Read the model definition and answer for the solid it produces. Units are mm, in the model's axes. A direction names the side the tool comes from. Coordinates: 2 decimals unless noted, no trailing zeros. Write each loop counter-clockwise with the first axis right and the second up, starting at its lowest first coordinate (ties: lowest second). Pieces come first, ordered by that corner, then holes. Notation, with made-up numbers: (67, 17.5) -> (119, 17.5) arc R10 ccw to (119, 31.5) -> close; hole circle Ø4 at (87.25, 79). An arc over 180 degrees is marked (long way). Use CSV: the item, a comma, the result in double quotes.
from build123d import *

# Parameters (mm, degrees)
F1_DEPTH = 5
F3_DEPTH = 2
F5_R     = 4.0386
F6_DEPTH = 2


with BuildPart() as f1:
    # F0 (on Top) → F1 (new body)
    with BuildSketch(Plane.XY):
        with BuildLine():
            ThreePointArc((-26.651348, 17.408332), (-28.98701, 16.85103), (-31.313855, 16.257994))
            Line((-31.313855, 16.257994), (-31.313855, -1.454417))
            ThreePointArc((-31.313855, -1.454417), (-29.445548, -2.127472), (-27.565881, -2.768118))
            Line((-27.565881, -2.768118), (-27.565881, 8.0386))
            Line((-27.565881, 8.0386), (-23.981268, -3.890644))
            ThreePointArc((-23.981268, -3.890644), (-21.785328, -4.515397), (-19.577401, -5.096367))
            Line((-19.577401, -5.096367), (-19.580996, 18.867471))
            ThreePointArc((-19.580996, 18.867471), (-21.536505, 18.497823), (-23.48716, 18.103362))
            Line((-23.48716, 18.103362), (-23.48716, 7.049417))
            Line((-23.48716, 7.049417), (-26.651348, 17.408332))
        make_face()
        with BuildLine():
            Line((48.388597, -1.454417), (48.388597, 16.257994))
            ThreePointArc((48.388597, 16.257994), (46.258605, 16.802327), (44.121183, 17.316716))
            Line((44.121183, 17.316716), (44.121183, 7.543997))
            Line((44.121183, 7.543997), (40.767098, 18.060365))
            ThreePointArc((40.767098, 18.060365), (38.40477, 18.538069), (36.035373, 18.979372))
            Line((36.035373, 18.979372), (36.035373, -5.250303))
            ThreePointArc((36.035373, -5.250303), (38.374392, -4.647226), (40.700207, -3.995081))
            Line((40.700207, -3.995081), (40.700207, 7.247278))
            Line((40.700207, 7.247278), (43.522989, -3.131948))
            ThreePointArc((43.522989, -3.131948), (45.965192, -2.320446), (48.388597, -1.454417))
        make_face()
        with BuildLine():
            ThreePointArc((-7.551971, 20.583244), (-12.343521, 20.013793), (-17.11526, 19.297039))
            Line((-17.11526, 19.297039), (-17.11526, -5.68932))
            ThreePointArc((-17.11526, -5.68932), (-12.30462, -6.684076), (-7.455836, -7.472168))
            Line((-7.455836, -7.472168), (-7.455836, -1.852502))
            Line((-7.455836, -1.852502), (-12.389002, -1.852502))
            Line((-12.389002, -1.852502), (-12.389002, 4.576681))
            Line((-12.389002, 4.576681), (-8.332584, 4.576681))
            Line((-8.332584, 4.576681), (-8.332584, 9.522207))
            Line((-8.332584, 9.522207), (-12.685815, 9.522207))
            Line((-12.685815, 9.522207), (-12.685815, 15.061192))
            Line((-12.685815, 15.061192), (-7.455836, 15.061192))
            Line((-7.455836, 15.061192), (-7.455836, 19.935173))
            Line((-7.455836, 19.935173), (-7.551971, 20.583244))
        make_face()
        with BuildLine():
            ThreePointArc((-7.455836, 20.59314), (-7.503905, 20.5882), (-7.551971, 20.583244))
            Line((-7.551971, 20.583244), (-7.455836, 19.935173))
            Line((-7.455836, 19.935173), (-7.455836, 20.59314))
        make_face()
        with BuildLine():
            Line((-7.455836, 20.59314), (-7.455836, 19.935173))
            Line((-7.455836, 19.935173), (-3.31518, -7.978035))
            ThreePointArc((-3.31518, -7.978035), (-0.89273, -8.203509), (1.533954, -8.377611))
            Line((1.533954, -8.377611), (2.747888, 8.928744))
            Line((2.747888, 8.928744), (4.034133, -8.503044))
            ThreePointArc((4.034133, -8.503044), (6.507916, -8.573444), (8.982641, -8.590516))
            Line((8.982641, -8.590516), (11.160356, 15.061197))
            Line((11.160356, 15.061197), (14.525345, 15.061197))
            Line((14.525345, 15.061197), (14.525345, -8.435146))
            ThreePointArc((14.525345, -8.435146), (16.803292, -8.293483), (19.077973, -8.106573))
            Line((19.077973, -8.106573), (19.077973, 15.061197))
            Line((19.077973, 15.061197), (22.041207, 15.061197))
            Line((22.041207, 15.061197), (22.041207, 20.828562))
            ThreePointArc((22.041207, 20.828562), (15.07889, 21.275037), (8.103599, 21.411077))
            Line((8.103599, 21.411077), (6.607726, 4.181039))
            Line((6.607726, 4.181039), (5.123083, 21.374465))
            ThreePointArc((5.123083, 21.374465), (2.93767, 21.311562), (0.753347, 21.218165))
            Line((0.753347, 21.218165), (-0.815041, 4.27995))
            Line((-0.815041, 4.27995), (-2.410396, 21.028664))
            ThreePointArc((-2.410396, 21.028664), (-4.934876, 20.831292), (-7.455836, 20.59314))
        make_face()
        with BuildLine():
            ThreePointArc((25.337448, 20.50822), (23.613483, 17.75595), (23.011211, 14.564663))
            Line((23.011211, 14.564663), (23.011211, -3.039429))
            ThreePointArc((23.011211, -3.039429), (24.095706, -5.410003), (25.924952, -7.267315))
            ThreePointArc((25.924952, -7.267315), (28.678591, -7.296316), (31.254217, -6.321887))
            ThreePointArc((31.254217, -6.321887), (33.502257, -4.16289), (34.178704, -1.120298))
            Line((34.178704, -1.120298), (34.178704, 14.564663))
            ThreePointArc((34.178704, 14.564663), (32.97203, 18.250105), (29.81934, 20.50822))
            ThreePointArc((29.81934, 20.50822), (27.578394, 20.977344), (25.337448, 20.50822))
        make_face()
        with BuildLine():
            Line((27.094735, -1.268663), (27.094735, 14.564663))
            ThreePointArc((27.094735, 14.564663), (28.506575, 15.976503), (29.918415, 14.564663))
            Line((29.918415, 14.564663), (29.918415, 0))
            ThreePointArc((29.918415, 0), (29.647931, -1.410752), (28.513743, -2.292226))
            ThreePointArc((28.513743, -2.292226), (27.542368, -2.143487), (27.094735, -1.268663))
        make_face(mode=Mode.SUBTRACT)
    extrude(amount=F1_DEPTH)


with BuildPart() as f3:
    # F2 (on Top) → F3 (new body)
    with BuildSketch(Plane.XY):
        with BuildLine():
            ThreePointArc((51.958822, 18.827472), (8.400722, 25.06269), (-35.087429, 18.356971))
            Line((-35.087429, 18.356971), (-35.087429, -5.168048))
            ThreePointArc((-35.087429, -5.168048), (8.499812, -11.534627), (51.958822, -4.344672))
            Line((51.958822, -4.344672), (51.958822, 18.827472))
        make_face()
    extrude(amount=-F3_DEPTH)


with BuildPart() as f1_1:
    add(f1.part)

    # F4: union F3
    add(f3.part)

    # F5 (on face) → F6 (join)
    with BuildSketch(Plane.XY):
        with BuildLine():
            Line((51.958822, 15.3059), (51.958822, 7.2414))
            Line((51.958822, 7.2414), (51.958822, -0.8231))
            Line((51.958822, -0.8231), (61.737822, -0.8231))
            ThreePointArc((61.737822, -0.8231), (66.22795, 1.036772), (68.087822, 5.5269))
            Line((68.087822, 5.5269), (68.087822, 8.9559))
            ThreePointArc((68.087822, 8.9559), (66.22795, 13.446028), (61.737822, 15.3059))
            Line((61.737822, 15.3059), (51.958822, 15.3059))
        make_face()
        with Locations((59.165195, 7.2414)):
            Circle(F5_R, mode=Mode.SUBTRACT)
    extrude(amount=-F6_DEPTH)


solid = f1_1.part
1. Each of these flat-tipped pins is pushed along its axis until it touches: pin 1 Ø7.5 at (x, y) = (59.17, 7.24) entering from -Z; pin 2 Ø0.9 at (x, y) = (29, 6) entering from +Z; pin 3 Ø2.5 at (y, z) = (6.5, 3.5) entering from +X; pin 4 Ø1.5 at (x, z) = (-10.5, 3.5) entering from -Y. Where does it stop, or does it pass through?
Solutions:
pin 1,"passes through"
pin 2,"stops at z = 0"
pin 3,"stops at x = 48.39"
pin 4,"stops at y = -7.13"
2. A cutting plane is placed at C-C (x = -6.5). Give the vertices of the cut face in (y, z).
Solutions:
outline,"(-10.89, -2) -> (24.24, -2) -> (24.24, 0) -> (20.69, 0) -> (20.69, 5) -> (13.49, 5) -> (13.49, 0) -> (-10.89, 0) -> close"
3. For a pull along Y with two mould halves and no side action, classify faces 1 (the cylindrical face through (28.64, -7.303, 2.465)), 2 (the flat face through (-10, 9.522, 2)), 3 (the cylindrical face through (2.968, 21.313, 2.465)) as pulls with the +Y half, pulls with the -Y half, needs draft (parallel to the pull), parting line crosses it, or undercut.
Solutions:
face 1,"pulls with the -Y half"
face 2,"undercut"
face 3,"pulls with the +Y half"
4. A cutting plane is placed at B-B (x = 46). Give the vertices of the cut face in (y, z), and give its area (3 significant figures).
Solutions:
outline,"(-6.17, -2) -> (20.47, -2) -> (20.47, 0) -> (16.87, 0) -> (16.87, 5) -> (-2.31, 5) -> (-2.31, 0) -> (-6.17, 0) -> close"
area,"149 mm^2"
5. A tool of negligible diameter and unlimited length cuts with its end or side. For faces 4 (the flat face through (23.011, 6, 2)), 5 (the flat face through (-12.686, 12, 2)), 6 (the cylindrical face through (-4.9, 20.834, 2.465)), from which of +Z, -Z, +X, -X, +Y, -Y can it reach the whole face along a straight path? Write none if from no direction.
Solutions:
face 4,"+Z, +Y, -Y"
face 5,"+Z"
face 6,"+Z, -X, +Y"
6. A cutting plane is placed at A-A (z = 2.75). Give the number of separate pieces and of enclosed holes in the cut face, and give its area (3 significant figures).
Solutions:
separate pieces,"4"
enclosed holes,"1"
area,"1,430 mm^2"
7. Find the intervals of material crossed by line 1 along Z through (x, y) = (56, 13.5); line 2 along Y through (x, z) = (58.5, -1.5); line 3 along Y through (x, z) = (38.5, -0.5), in increasing order.
Solutions:
line 1,"z = -2 to 0"
line 2,"y = -0.82 to 3.26, 11.22 to 15.31"
line 3,"y = -8.06 to 22.17"
